For this review, take the finished solid that the model builds, in its own axes (mm). A direction names the side the tool comes from. Give positions to 0.01 mm unless a question says otherwise; leave off trailing zeros. Loops run counter-clockwise (first coordinate to the right, second up) from the corner with the lowest first, then second, coordinate; pieces in that order, holes last.
Autodesk Fusion 360 part; units mm, degrees
sketch "Sketch1" plane through (0, 0, 0) normal (0, 0, 1) x (1, 0, 0)
  line L0 (0, 0) -> (174, 0)
  line L1 (174, 0) -> (174, 109)
  line L2 (174, 109) -> (0, 109)
  line L3 (0, 109) -> (0, 0)
  dimension "d1" = 174
  dimension "d2" = 109
extrude "Extrude1" add sketch "Sketch1" along normal blind 2
sketch "Sketch2" plane through (0, 0, 2) normal (0, 0, 1) x (-1, 0, 0)
  line L0 (0, -109) -> (0, 0)
  line L1 (0, 0) -> (-174, 0)
  line L2 (-174, 0) -> (-174, -109)
  line L3 (-174, -109) -> (0, -109)
  point P0 (-3.5, -3.5)
  point P1 (-3.5, -105.5)
  point P2 (-170.5, -105.5)
  point P3 (-170.5, -3.5)
hole "Hole1" at (170.5, 3.5, 2) at (3.5, 105.5, 2) at (3.5, 3.5, 2) at (170.5, 105.5, 2) direction (0, 0, -1) diameter 3.4 depth 6 tip angle 180 countersink diameter 5.75 countersink angle 90
sketch "Sketch5" plane through (0, 0, 2) normal (0, 0, 1) x (-1, 0, 0)
  circle A0 centre (-3.5, -3.5) radius 2.875
  circle A1 centre (-170.5, -3.5) radius 2.875
  circle A2 centre (-3.5, -105.5) radius 2.875
  circle A3 centre (-170.5, -105.5) radius 2.875
  line L0 (0, -109) -> (0, 0)
  line L1 (0, 0) -> (-174, 0)
  line L2 (-174, 0) -> (-174, -109)
  line L3 (-174, -109) -> (0, -109)
  line L4 (-10, -10) -> (-100, -100)
  line L5 (-100, -100) -> (-103.5355, -96.4645)
  line L6 (-103.5355, -96.4645) -> (-13.5355, -6.4645)
  line L7 (-13.5355, -6.4645) -> (-10, -10)
  line L8 (-30, -10) -> (-120, -100)
  line L9 (-123.5355, -96.4645) -> (-33.5355, -6.4645)
  line L10 (-33.5355, -6.4645) -> (-30, -10)
  line L11 (-120, -100) -> (-123.5355, -96.4645)
  line L12 (-50, -10) -> (-140, -100)
  line L13 (-143.5355, -96.4645) -> (-53.5355, -6.4645)
  line L14 (-53.5355, -6.4645) -> (-50, -10)
  line L15 (-140, -100) -> (-143.5355, -96.4645)
  line L16 (-70, -10) -> (-160, -100)
  line L17 (-163.5355, -96.4645) -> (-73.5355, -6.4645)
  line L18 (-73.5355, -6.4645) -> (-70, -10)
  line L19 (-160, -100) -> (-163.5355, -96.4645)
  dimension "d17" = 5
  dimension "d20" = -60
  dimension "d21" = 0
extrude "Extrude2" cut sketch "Sketch5" against normal blind 40 contours L4 L5 L6 L7 | L8 L9 L10 L11 | L12 L13 L14 L15 | L16 L17 L18 L19
Item 1: The part is to be moulded in two halves that separate along Y. For faces 1 (the flat face through (114, 54, 1)), 2 (the flat face through (86, 55, 0)), say which applies: released by +Y, released by -Y, zero draft, split by the parting line, or undercut.
Answer:
face 1: undercut
face 2: zero draft
Item 2: Clearance check with flat-ended pins moving along their axes: pin 1 Ø2 at (x, y) = (45.5, 95.5) entering from -Z; pin 2 Ø4 at (x, y) = (3.5, 3.5) entering from +Z (3 decimals). State where each tip first meets the part, or that it passes through.
Answer:
pin 1: stops at z = 0
pin 2: stops at z = 1.125
Item 3: Take a section at D-D on x = 78. Give the boundary of the cut face in (y, z).
Answer:
outline: (0, 0) - (10.93, 0) - (10.93, 2) - (0, 2) - close; (18, 0) - (30.93, 0) - (30.93, 2) - (18, 2) - close; (38, 0) - (50.93, 0) - (50.93, 2) - (38, 2) - close; (58, 0) - (70.93, 0) - (70.93, 2) - (58, 2) - close; (78, 0) - (109, 0) - (109, 2) - (78, 2) - close
Item 4: Take a section at B-B on x = 3.5. Give the boundary of the cut face in (y, z) (3 decimals).
Answer:
outline: (0, 0) - (1.8, 0) - (1.8, 0.825) - (0.625, 2) - (0, 2) - close; (5.2, 0) - (103.8, 0) - (103.8, 0.825) - (102.625, 2) - (6.375, 2) - (5.2, 0.825) - close; (107.2, 0) - (109, 0) - (109, 2) - (108.375, 2) - (107.2, 0.825) - close
Item 5: Take a section at C-C on y = 77. Give the boundary of the cut face in (x, z), and give its area (3 significant figures).
Answer:
outline: (0, 0) - (77, 0) - (77, 2) - (0, 2) - close; (84.07, 0) - (97, 0) - (97, 2) - (84.07, 2) - close; (104.07, 0) - (117, 0) - (117, 2) - (104.07, 2) - close; (124.07, 0) - (137, 0) - (137, 2) - (124.07, 2) - close; (144.07, 0) - (174, 0) - (174, 2) - (144.07, 2) - close
area: 291 mm2
Item 6: For L1, parallel to Y at x = 3.5, z = 0.35; L2, parallel to X at y = 105.5, z = 0.55; L3, parallel to X at y = 25, z = 0.55, list the stretches that pass through material, from the lowest coordinate up.
Answer:
L1: y = 0 to 1.8, 5.2 to 103.8, 107.2 to 109
L2: x = 0 to 1.8, 5.2 to 168.8, 172.2 to 174
L3: x = 0 to 25, 32.07 to 45, 52.07 to 65, 72.07 to 85, 92.07 to 174
Item 7: Tool access review of faces 3 (the flat face through (119.166, 52.094, 1.014)), 4 (the flat face through (86, 55, 2)): name each direction out of +Z, -Z, +X, -X, +Y, -Y from which nothing blocks a thin tool from reaching the whole face with its end or side.
Answer:
face 3: +Z, -Z
face 4: +Z, +X, -X, +Y, -Y
Item 8: Take a section at A-A on y = 105.5. Give the boundary of the cut face in (x, z) (3 decimals).
Answer:
outline: (0, 0) - (1.8, 0) - (1.8, 0.825) - (0.625, 2) - (0, 2) - close; (5.2, 0) - (168.8, 0) - (168.8, 0.825) - (167.625, 2) - (6.375, 2) - (5.2, 0.825) - close; (172.2, 0) - (174, 0) - (174, 2) - (173.375, 2) - (172.2, 0.825) - close
